Read the model definition and answer for the solid it produces. Units are mm, in the model's axes. Face numbers are marked on the shaded views. A direction names the side the tool comes from. Coordinates: 2 decimals unless noted, no trailing zeros. Write each loop counter-clockwise with the first axis right and the second up, starting at its lowest first coordinate (ties: lowest second). Pieces come first, ordered by that corner, then holes. Notation, with made-up numbers: M -15.5,79 L -3.5,79 A30 ccw -3.5,104 Z; hole C 50.25,20 d8. An arc over 180 degrees is marked long. Use a Markdown table: item, result. Add a question column.
from build123d import *

# Parameters (mm, degrees)
F0_W     = 80
F0_H     = 80
F0_R     = 2.5
F0_R_2   = 15
F1_DEPTH = 6
F2_W     = 60
F2_H     = 2
F2_H_2   = 4
F3_DEPTH = 40
F4_R     = 3
F5_DEPTH = 6
F6_W     = 80
F6_H     = 4
F7_DEPTH = 6


with BuildPart() as f1:
    # F0 (on Front) → F1 (new body)
    with BuildSketch(Plane.XZ):
        Rectangle(F0_W, F0_H)
        with Locations((-34.8, -34.8)):
            Circle(F0_R, mode=Mode.SUBTRACT)
        with Locations((34.8, -34.8)):
            Circle(F0_R, mode=Mode.SUBTRACT)
        with Locations((-34.8, 34.8)):
            Circle(F0_R, mode=Mode.SUBTRACT)
        Circle(F0_R_2, mode=Mode.SUBTRACT)
        with Locations((34.8, 34.8)):
            Circle(F0_R, mode=Mode.SUBTRACT)
    extrude(amount=F1_DEPTH)

    # F2 (on face) → F3 (join)
    with BuildSketch(Plane.XZ.offset(6)):
        with Locations((0, -39)):
            Rectangle(F2_W, F2_H)
        with Locations((0, -42)):
            Rectangle(F2_W, F2_H_2)
    extrude(amount=F3_DEPTH)

    # F4 (on face) → F5 (cut, through all)
    with BuildSketch(Plane.XY.offset(-38)):
        with Locations((-22, -38)):
            Circle(F4_R)
        with Locations((-22, -16)):
            Circle(F4_R)
        with Locations((22, -16)):
            Circle(F4_R)
        with Locations((22, -38)):
            Circle(F4_R)
    extrude(amount=-F5_DEPTH, mode=Mode.SUBTRACT)

    # F6 (on face) → F7 (join, through all)
    with BuildSketch(Plane.XZ.offset(6)):
        with Locations((0, -42)):
            Rectangle(F6_W, F6_H)
    extrude(amount=-F7_DEPTH)


solid = f1.part
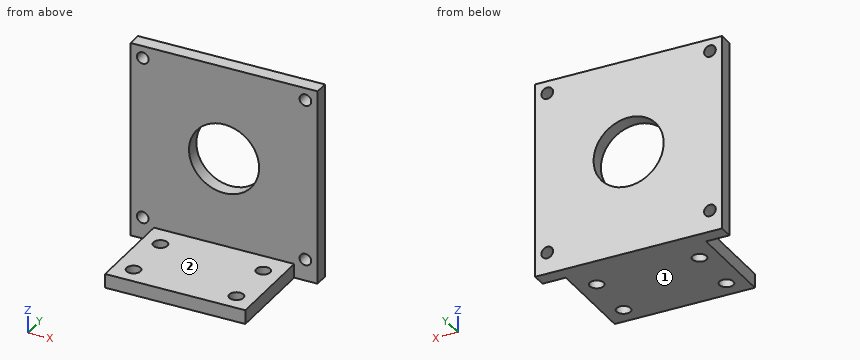
Item 1: For the marked faces 1 and 2, determine the directions among +Z, -Z, +X, -X, +Y, -Y from which every point of the face is accessible in a straight line to the end or side of a thin tool.
Item 2: Find section A-A on y = -16. Give the vertices of the cut face in (x, z).
Item 3: Each of these flat-tipped pins is pushed along its axis until it touches: pin 1 (4 mm diameter, centred on x = -34.8, z = 34.8, fed in from +Y); pin 2 (10 mm diameter, centred on x = -22, y = -34.5, fed in from +Z); pin 3 (24 mm diameter, centred on x = 13, z = -0.5, fed in from -Y); pin 4 (3 mm diameter, centred on y = -30, z = -40, fed in from -X). Where does it stop, or does it pass through?
Item 4: Consider probe 1 along Y at (x, z) = (22, -41.8); probe 2 along X at (y, z) = (-1, 34); probe 3 along Y at (x, z) = (-6, 36). Determine where each line is inside the solid, lowest interval first.
Item 5: Find section C-C on z = 9. Give the vertices of the cut face in (x, y), then the cut area to 3 significant figures.
Item 6: Find section B-B on x = 34.8. Give the vertices of the cut face in (y, z).
Item 7: Find section D-D on x = 6.5. Give the vertices of the cut face in (y, z).
Geometry says:
| question | item | result |
|---|---|---|
| 1 | face 1 | -Z, +X, -X, +Y, -Y |
| 1 | face 2 | +Z, +X, -X, -Y |
| 2 | outline | M -30,-44 L -25,-44 L -25,-38 L -30,-38 Z; M -19,-44 L 19,-44 L 19,-38 L -19,-38 Z; M 25,-44 L 30,-44 L 30,-38 L 25,-38 Z |
| 3 | pin 1 | passes through |
| 3 | pin 2 | stops at z = -38 |
| 3 | pin 3 | stops at y = -6 |
| 3 | pin 4 | stops at x = -30 |
| 4 | probe 1 | y = -46 to -41, -35 to -19, -13 to 0 |
| 4 | probe 2 | x = -40 to -37.17, -32.43 to 32.43, 37.17 to 40 |
| 4 | probe 3 | y = -6 to 0 |
| 5 | outline | M -40,-6 L -12,-6 L -12,0 L -40,0 Z; M 12,-6 L 40,-6 L 40,0 L 12,0 Z |
| 5 | area | 336 mm2 |
| 6 | outline | M -6,-44 L 0,-44 L 0,-37.3 L -6,-37.3 Z; M -6,-32.3 L 0,-32.3 L 0,32.3 L -6,32.3 Z; M -6,37.3 L 0,37.3 L 0,40 L -6,40 Z |
| 7 | outline | M -46,-44 L 0,-44 L 0,-13.52 L -6,-13.52 L -6,-38 L -46,-38 Z; M -6,13.52 L 0,13.52 L 0,40 L -6,40 Z |
